```python
from build123d import *

# Parameters (mm, degrees)
F0_W     = 50
F0_H     = 65
F1_DEPTH = 35
F2_T     = -2
F4_DEPTH = 100


with BuildPart() as f1:
    # F0 (on Top) → F1 (new body)
    with BuildSketch(Plane.XY):
        with Locations((25, -32.5)):
            Rectangle(F0_W, F0_H)
    extrude(amount=F1_DEPTH)

    # F2
    f2_openings = [f1.faces().sort_by_distance(p)[0] for p in [
        (25, -32.5, 35),
    ]]
    offset(amount=F2_T, openings=f2_openings)

    # F3 (on face) → F4 (cut, symmetric)
    with BuildSketch(Plane.XZ.offset(65)):
        with BuildLine():
            Line((35, 31.769874), (15, 31.769874))
            ThreePointArc((15, 31.769874), (13.153528, 29.923402), (15, 28.076929))
            Line((15, 28.076929), (35, 28.076929))
            ThreePointArc((35, 28.076929), (36.846472, 29.923402), (35, 31.769874))
        make_face()
    extrude(amount=F4_DEPTH, both=True, mode=Mode.SUBTRACT)


solid = f1.part
```
Geometry check sheet. Reference: the model listing, model coordinates, mm. A direction names the side the tool comes from. Give positions to 0.01 mm unless a question says otherwise; leave off trailing zeros. Order: outer loops, then holes, each group sorted by start corner. A loop starts at its lowest first (then second) coordinate and runs counter-clockwise, first axis right, second up.
1. Section check A-A, the plane x = 27. Enter the section's corners in (y, z).
2. Section check D-D, the plane x = 8.5. Enter the section's corners in (y, z).
3. Release check for a two-part mould opening along Z. For faces 1 (the face through (25, -32, 2)), 2 (the face through (13.154, -1.014, 29.964)), 3 (the face through (2, -33, 18)) record: pulls with the +Z half, pulls with the -Z half, needs draft (parallel to the pull), parting line crosses it, or undercut.
4. Gauge pin test, flat end, axial feed: pin 1 Ø6 at (x, y) = (14, -45) entering from +Z. Record the tip position at first contact, or that the pin passes through.
5. Thickness scan on L1, parallel to Y at x = 31.5, z = 13; L2, parallel to X at y = -6.5, z = 9; L3, parallel to Z at x = 45, y = -53. Record the ranges inside material, lowest first.
6. Section check C-C, the plane y = -59.5. Enter the section's corners in (x, z).
7. Section check B-B, the plane z = 20.5. Enter the section's corners in (x, y).
8. Access from +Z, -Z, +X, -X, +Y, -Y to the whole of each face (thin tool, end or side, straight path). Record for faces 4 (the face through (25, -65, 17)), 5 (the face through (25, -1, 28.077)), 6 (the face through (25, -2, 18)).
Values follow:
1. outline: (-65, 0) - (0, 0) - (0, 28.08) - (-2, 28.08) - (-2, 2) - (-63, 2) - (-63, 28.08) - (-65, 28.08) - close; (-65, 31.77) - (-63, 31.77) - (-63, 35) - (-65, 35) - close; (-2, 31.77) - (0, 31.77) - (0, 35) - (-2, 35) - close
2. outline: (-65, 0) - (0, 0) - (0, 35) - (-2, 35) - (-2, 2) - (-63, 2) - (-63, 35) - (-65, 35) - close
3. face 1: pulls with the +Z half
3. face 2: undercut
3. face 3: needs draft
4. pin 1: stops at z = 2
5. L1: y = -65 to -63, -2 to 0
5. L2: x = 0 to 2, 48 to 50
5. L3: z = 0 to 2
6. outline: (0, 0) - (50, 0) - (50, 35) - (48, 35) - (48, 2) - (2, 2) - (2, 35) - (0, 35) - close
7. outline: (0, -65) - (50, -65) - (50, 0) - (0, 0) - close; hole (2, -63) - (48, -63) - (48, -2) - (2, -2) - close
8. face 4: +Z, -Z, +X, -X, -Y
8. face 5: +Y, -Y
8. face 6: +Z
